from build123d import *

# Parameters (mm, degrees)
BOSS_EXTRUDE2_DEPTH      = 20
FILLET1_START            = -1
FILLET1_DEPTH            = 9
CUT_EXTRUDE2_REACH       = 31.394
CUT_EXTRUDE2_END_RADIUS  = 20
SKETCH4_R                = 2.5125
BOSS_EXTRUDE3_REACH      = 31.394
BOSS_EXTRUDE3_END_RADIUS = 16.3
SKETCH6_R                = 1.75
SKETCH7_R                = 4.65
CUT_EXTRUDE4_DEPTH       = 1


with BuildPart() as part:
    # Sketch3 → Boss-Extrude2 (new body)
    with BuildSketch(Plane(origin=(0, 0, 0), x_dir=(0, 0, -1), z_dir=(1, 0, 0))):
        with BuildLine():
            Line((0, 20), (-8, 20))
            Line((-8, 20), (-8, 0))
            Line((-8, 0), (0, 0))
            ThreePointArc((0, 0), (-2.679491924, 10), (0, 20))
        make_face()
    extrude(amount=BOSS_EXTRUDE2_DEPTH)

    # Fillet1: read off the stored shape, not the designer's step
    # Fillet1 outline → Fillet1 (cut)
    with BuildSketch(Plane.XY.offset(FILLET1_START)):
        with BuildLine():
            Line((0, 20), (0, 10))
            ThreePointArc((0, 10), (2.928932188, 17.071067812), (10, 20))
            Line((10, 20), (0, 20))
        make_face()
        with BuildLine():
            ThreePointArc((10, 0), (2.928932188, 2.928932188), (0, 10))
            Line((0, 10), (0, 0))
            Line((0, 0), (10, 0))
        make_face()
        with BuildLine():
            Line((20, 20), (10, 20))
            ThreePointArc((10, 20), (17.071067812, 17.071067812), (20, 10))
            Line((20, 10), (20, 20))
        make_face()
        with BuildLine():
            ThreePointArc((20, 10), (17.071067812, 2.928932188), (10, 0))
            Line((10, 0), (20, 0))
            Line((20, 0), (20, 10))
        make_face()
    extrude(amount=FILLET1_DEPTH, mode=Mode.SUBTRACT)

    # Cut-Extrude2: up to this cylinder (the profile starts outside it)
    cut_extrude2_end = Plane(origin=(10, 10, -17.320508076), z_dir=(-1, 0, 0)) * Cylinder(CUT_EXTRUDE2_END_RADIUS, 103.788, mode=Mode.PRIVATE)
    # Sketch4 → Cut-Extrude2 (cut, up to the surface)
    with BuildSketch(Plane.XY.offset(8), mode=Mode.PRIVATE) as cut_extrude2_sk1:
        with Locations((10, 10)):
            Circle(SKETCH4_R)
    cut_extrude2_tool1 = extrude(cut_extrude2_sk1.sketch, amount=-CUT_EXTRUDE2_REACH, mode=Mode.PRIVATE) - cut_extrude2_end
    add(cut_extrude2_tool1.solids().sort_by_distance((10, 10, 8))[0], mode=Mode.SUBTRACT)

    # Boss-Extrude3: up to this cylinder (the profile starts outside it)
    boss_extrude3_end = Plane(origin=(10, 10, -17.320508076), z_dir=(-1, 0, 0)) * Cylinder(BOSS_EXTRUDE3_END_RADIUS, 109.388, mode=Mode.PRIVATE)
    # Sketch6 → Boss-Extrude3 (add, up to the surface)
    with BuildSketch(Plane.XY.offset(8), mode=Mode.PRIVATE) as boss_extrude3_sk1:
        with Locations((3.5, 10)):
            Circle(SKETCH6_R)
    boss_extrude3_tool1 = extrude(boss_extrude3_sk1.sketch, amount=-BOSS_EXTRUDE3_REACH, mode=Mode.PRIVATE) - boss_extrude3_end
    add(boss_extrude3_tool1.solids().sort_by_distance((3.5, 10, 8))[0])
    # Sketch6 → Boss-Extrude3 (add, up to the surface)
    with BuildSketch(Plane.XY.offset(8), mode=Mode.PRIVATE) as boss_extrude3_sk2:
        with Locations((16.5, 10)):
            Circle(SKETCH6_R)
    boss_extrude3_tool2 = extrude(boss_extrude3_sk2.sketch, amount=-BOSS_EXTRUDE3_REACH, mode=Mode.PRIVATE) - boss_extrude3_end
    add(boss_extrude3_tool2.solids().sort_by_distance((16.5, 10, 8))[0])

    # Sketch7 → Cut-Extrude4 (cut)
    with BuildSketch(Plane.XY.offset(8)):
        with Locations((10, 10)):
            Circle(SKETCH7_R)
    extrude(amount=-CUT_EXTRUDE4_DEPTH, mode=Mode.SUBTRACT)


solid = part.part
The listing builds one solid part. Answer for the finished solid, in the listing's coordinates (mm). A direction names the side the tool comes from. Give positions to 0.01 mm unless a question says otherwise; leave off trailing zeros. Order: outer loops, then holes, each group sorted by start corner. A loop starts at its lowest first (then second) coordinate and runs counter-clockwise, first axis right, second up. Notation, with made-up numbers: (21, 5) - (34, 5) arc R20 cw to (34, 29) - close; hole circle Ø8 at (86, -27). An arc over 180 degrees is marked (long way). Use one line per item in the form item = value.
1) Each of these flat-tipped pins is pushed along its axis until it touches: pin 1 (1.5 mm diameter, centred on y = 8, z = 6, fed in from -X); pin 2 (4 mm diameter, centred on x = 15, z = 7, fed in from +Y); pin 3 (3 mm diameter, centred on y = 3.5, z = 2.5, fed in from +X); pin 4 (4.5 mm diameter, centred on x = 10, y = 10, fed in from -Z). Where does it stop, or does it pass through?
Verdict:
pin_1 = 0.08
pin_2 = 19.54
pin_3 = 18.66
pin_4 = through
2) Find section A-A on z = 1. Determine the outline of the cut face in (x, y).
Verdict:
outline = circle Ø3.5 at (3.5, 10); (4.03, 1.98) arc R10 ccw to (15.97, 1.98) - close; (4.03, 18.02) - (15.97, 18.02) arc R10 ccw to start; circle Ø3.5 at (16.5, 10)
3) Consider probe 1 along Y at (x, z) = (10, 7.6); probe 2 along Y at (x, z) = (10, 6.05); probe 3 along X at (y, z) = (13, 7.25). Determine where each line is inside the solid, lowest interval first. Write a range as [from, to].
Verdict:
probe_1 = [0, 5.35], [14.65, 20]
probe_2 = [0, 7.49], [12.51, 20]
probe_3 = [0.46, 6.45], [13.55, 19.54]
4) For faces 3 (the cylindrical face through (8.99, 5.46, 7.51)), 4 (the cylindrical face through (3.272, 11.735, 0.809)), 5 (the cylindrical face through (3.47, 9.97, -1.02)), determine the directions among +Z, -Z, +X, -X, +Y, -Y from which every point of the face is accessible in a straight line to the end or side of a thin tool.
Verdict:
face_3 = +Z
face_4 = -Z
face_5 = -Z, +X, -X
5) Find section D-D on x = 8.25. Determine the outline of the cut face in (y, z).
Verdict:
outline = (0.15, 0.09) arc R20 cw to (8.2, 2.6) - (8.2, 7) - (5.69, 7) - (5.69, 8) - (0.15, 8) - close; (11.8, 2.6) arc R20 cw to (19.85, 0.09) - (19.85, 8) - (14.31, 8) - (14.31, 7) - (11.8, 7) - close
6) Find section B-B on z = 4.75. Determine the outline of the cut face in (x, y) (1 decimal), and give its area (3 significant figures).
Verdict:
outline = circle Ø20 at (10, 10); hole circle Ø5 at (10, 10)
area = 294 mm^2
7) The mould has two halves that part along Y. Classify faces 1 (the flat face through (7.6, 5.7, 8)), 2 (the cylindrical face through (16.47, 9.97, -1.02)): released by +Y, released by -Y, zero draft, split by the parting line, or undercut.
Verdict:
face_1 = zero draft
face_2 = undercut
8) Find section C-C on y = 9. Determine the outline of the cut face in (x, z), and give its area (3 significant figures).
Verdict:
outline = (0.05, 2.65) - (2.06, 2.65) - (2.06, -1.05) - (4.94, -1.05) - (4.94, 2.65) - (7.7, 2.65) - (7.7, 7) - (5.46, 7) - (5.46, 8) - (0.05, 8) - close; (12.3, 2.65) - (15.06, 2.65) - (15.06, -1.05) - (17.94, -1.05) - (17.94, 2.65) - (19.95, 2.65) - (19.95, 8) - (14.54, 8) - (14.54, 7) - (12.3, 7) - close
area = 98.5 mm^2
